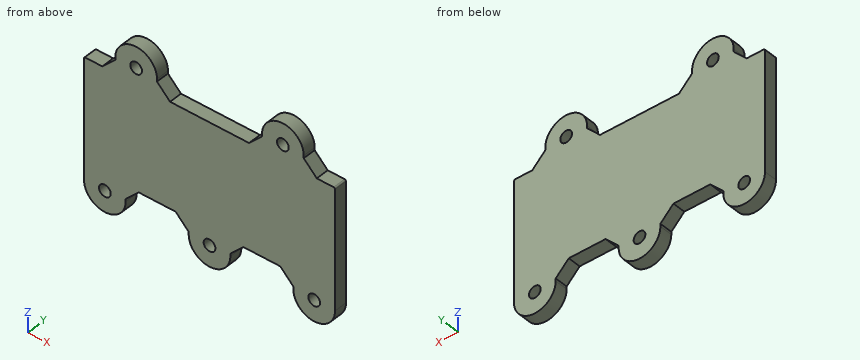
```python
from build123d import *

# Parameters (mm, degrees)
BOSS_EXTRUDE1_DEPTH  = 5
CHAMFER1_SIZE        = 5
M4_CLEARANCE_HOLE1_D = 4.5
FILLET1_R            = 0.5


with BuildPart() as part:
    # Sketch1 → Boss-Extrude1 (new body)
    with BuildSketch(Plane(origin=(0, 0, 0), x_dir=(1, 0, 0), z_dir=(0, 1, 0))):
        with BuildLine():
            Line((48.15, -20.05), (48.15, 20.05))
            Line((48.15, 20.05), (48.15, 26.05))
            ThreePointArc((48.15, 26.05), (40.15, 34.05), (32.15, 26.05))
            Line((32.15, 26.05), (32.15, 20.05))
            Line((32.15, 20.05), (8, 20.05))
            Line((8, 20.05), (8, 26.05))
            ThreePointArc((8, 26.05), (0, 34.05), (-8, 26.05))
            Line((-8, 26.05), (-8, 20.05))
            Line((-8, 20.05), (-32.15, 20.05))
            Line((-32.15, 20.05), (-32.15, 26.05))
            ThreePointArc((-32.15, 26.05), (-40.15, 34.05), (-48.15, 26.05))
            Line((-48.15, 26.05), (-48.15, 20.05))
            Line((-48.15, 20.05), (-48.15, -20.05))
            Line((-48.15, -20.05), (-36.15, -20.05))
            Line((-36.15, -20.05), (-36.15, -26.05))
            ThreePointArc((-36.15, -26.05), (-28.15, -34.05), (-20.15, -26.05))
            Line((-20.15, -26.05), (-20.15, -20.05))
            Line((-20.15, -20.05), (20.15, -20.05))
            Line((20.15, -20.05), (20.15, -26.05))
            ThreePointArc((20.15, -26.05), (28.15, -34.05), (36.15, -26.05))
            Line((36.15, -26.05), (36.15, -20.05))
            Line((36.15, -20.05), (48.15, -20.05))
        make_face()
    extrude(amount=BOSS_EXTRUDE1_DEPTH)

    # Chamfer1
    chamfer1_edges = [part.edges().sort_by_distance(p)[0] for p in [
        (36.15, 2.5, 20.05),
        (20.15, 2.5, 20.05),
        (-20.15, 2.5, 20.05),
        (-36.15, 2.5, 20.05),
        (-32.15, 2.5, -20.05),
        (-8, 2.5, -20.05),
        (8, 2.5, -20.05),
        (32.15, 2.5, -20.05),
    ]]
    chamfer(chamfer1_edges, length=CHAMFER1_SIZE)

    # M4 Clearance Hole1 (through all)
    with Locations(Plane(origin=(28.15, 0, 26.05), x_dir=(0, 0, -1), z_dir=(0, -1, 0))):
        with Locations((0, 0), (52.1, -68.3), (52.1, -28.15), (52.1, 12), (0, -56.3)):
            Hole(M4_CLEARANCE_HOLE1_D / 2)

    # Fillet1
    fillet1_edges = [part.edges().sort_by_distance(p)[0] for p in [
        (-48.15, 2.5, 20.05),
        (48.15, 2.5, 20.05),
    ]]
    fillet(fillet1_edges, radius=FILLET1_R)


solid = part.part
```
Input: part model. Units: mm. Frame: model coordinates. Coordinates: 2 decimals unless noted, no trailing zeros. Loops run counter-clockwise (first coordinate to the right, second up) from the corner with the lowest first, then second, coordinate; pieces in that order, holes last. Notation, with made-up numbers: M 59.25,65.25 L 74.25,65.25 A24 ccw 74.25,103.25 Z; hole C 21.5,6 d8. An arc over 180 degrees is marked long. One line per item, written item: value.
(1) Line query: line 1 along X through (y, z) = (1.8, -26.05); line 2 along X through (y, z) = (2.3, 26.05); line 3 along X through (y, z) = (1.95, -23). Output: solid intervals per line, ascending. Write a range as from..to.
Filled in:
line 1: -48.15..-42.4, -37.9..-32.15, -8..-2.25, 2.25..8, 32.15..37.9, 42.4..48.15
line 2: -36.15..-30.4, -25.9..-20.15, 20.15..25.9, 30.4..36.15
line 3: -48.15..-30.1, -10.05..10.05, 30.1..48.15
(2) Section C-C (y = 3.7). Give the number of separate pieces and of enclosed holes in the cut face, and give its area (3 significant figures).
Filled in:
separate pieces: 1
enclosed holes: 5
area: 4,860 mm^2
(3) Section D-D (x = -17.5). Output: boundary loops of the cut face in (y, z), and give its area (3 significant figures).
Filled in:
outline: M 0,-20.05 L 5,-20.05 L 5,22.4 L 0,22.4 Z
area: 212 mm^2
(4) Pin query (flat end, axial travel): pin 1 (2.5 mm diameter, centred on x = 0, z = -26.05, fed in from +Y); pin 2 (0.5 mm diameter, centred on y = 3.5, z = 25.5, fed in from -X); pin 3 (1.5 mm diameter, centred on x = -44.5, y = 3.5, fed in from +Z); pin 4 (1.5 mm diameter, centred on x = -22, y = 3.5, fed in from -Z). Return the tip coordinate at first contact, or that it passes through.
Filled in:
pin 1: through
pin 2: x = -36.15
pin 3: z = 20.05
pin 4: z = -20.05
(5) Section B-B (z = 30.5). Output: boundary loops of the cut face in (x, y), and give its area (3 significant figures).
Filled in:
outline: M -34.8,0 L -21.5,0 L -21.5,5 L -34.8,5 Z; M 21.5,0 L 34.8,0 L 34.8,5 L 21.5,5 Z
area: 133 mm^2
(6) Section A-A (x = 28.15). Output: boundary loops of the cut face in (y, z).
Filled in:
outline: M 0,-21.05 L 5,-21.05 L 5,23.8 L 0,23.8 Z; M 0,28.3 L 5,28.3 L 5,34.05 L 0,34.05 Z
